For this review, take the finished solid that the model builds, in its own axes (mm). A direction names the side the tool comes from. Give positions to 0.01 mm unless a question says otherwise; leave off trailing zeros. Write each loop counter-clockwise with the first axis right and the second up, starting at its lowest first coordinate (ties: lowest second). Pieces come first, ordered by that corner, then holes.
from build123d import *

# Parameters (mm, degrees)
F0_W     = 150
F0_H     = 70
F1_DEPTH = 100
F2_T     = -5


# Not quite as in the source:
# - the program builds the solid bodies; features that only make, move or delete a surface that nothing else refers to are left out


with BuildPart() as f1:
    # F0 (on Top) → F1 (new body)
    with BuildSketch(Plane.XY):
        Rectangle(F0_W, F0_H)
    extrude(amount=F1_DEPTH)

    # F2
    f2_openings = [f1.faces().sort_by_distance(p)[0] for p in [
        (0, 0, 100),
    ]]
    offset(amount=F2_T, openings=f2_openings)


solid = f1.part
(1) Clearance check with a flat-ended pin moving along its axis: pin 1 Ø8 at (x, y) = (32, -27) entering from +Z. State where the tip first meets the part, or that it passes through.
(2) The part is to be moulded in two halves that separate along X. For faces 3 (the flat face through (-1, -30, 52)), 4 (the flat face through (-1, -35, 49)), 5 (the flat face through (-75, 0, 49)), say which applies: +X half, -X half, draft (parallel to the pull), parting line (faces both ways), or undercut.
(3) Tool access review of faces 1 (the flat face through (-1, 0, 5)), 2 (the flat face through (-1, 35, 49)): name each direction out of +Z, -Z, +X, -X, +Y, -Y from which nothing blocks a thin tool from reaching the whole face with its end or side.
(4) For L1, parallel to X at y = -13, z = 5.5; L2, parallel to Y at x = 32, z = 74; L3, parallel to Z at x = -64, y = -1.5, list the stretches that pass through material, from the lowest coordinate up.
(5) We need section B-B (y = -7.5). Write out the cut boundary in (x, z), and give its area (3 significant figures).
(6) We need section A-A (z = 18). Write out the cut boundary in (x, y).
(7) We need section C-C (x = 4.5). Write out the cut boundary in (y, z).
The answers:
1. pin 1: stops at z = 100
2. face 3: undercut
2. face 4: draft
2. face 5: -X half
3. face 1: +Z
3. face 2: +Z, -Z, +X, -X, +Y
4. L1: x = -75 to -70, 70 to 75
4. L2: y = -35 to -30, 30 to 35
4. L3: z = 0 to 5
5. outline: (-75, 0) - (75, 0) - (75, 100) - (70, 100) - (70, 5) - (-70, 5) - (-70, 100) - (-75, 100) - close
5. area: 1,700 mm2
6. outline: (-75, -35) - (75, -35) - (75, 35) - (-75, 35) - close; hole (-70, -30) - (70, -30) - (70, 30) - (-70, 30) - close
7. outline: (-35, 0) - (35, 0) - (35, 100) - (30, 100) - (30, 5) - (-30, 5) - (-30, 100) - (-35, 100) - close
